Part model, mm, in its own coordinate system. Face numbers are marked on the shaded views. A direction names the side the tool comes from. Coordinates: 2 decimals unless noted, no trailing zeros. Order: outer loops, then holes, each group sorted by start corner. A loop starts at its lowest first (then second) coordinate and runs counter-clockwise, first axis right, second up. Notation, with made-up numbers: (-37, -12.5) - (4, -12.5) arc R29 cw to (4, 7.5) - close; hole circle Ø10 at (-3, 30.5). An arc over 180 degrees is marked (long way). Use a Markdown table: item, result. Add a question column.
1) Saw through at B-B on z = 0. List the corners of the cut face in (x, y), then the cut area to 3 significant figures.
2) Saw through at C-C on y = 12. List the corners of the cut face in (x, z), then the cut area to 3 significant figures.
3) Wall check: L1, parallel to Z at x = 0.1, y = 4; L2, parallel to X at y = 17, z = 2; L3, parallel to Y at x = -21.5, z = -4.5. Give the ranges that are in metal, low to high. Write a range as [from, to].
4) Tool access for the marked faces 1 and 2: list every direction of +Z, -Z, +X, -X, +Y, -Y with a clear straight run to the whole face (end or side of a thin tool).
5) Drop flat-ended pins along their axis: P1, Ø5, axis at x = -13, z = 0, coming from the -Y side; P2, Ø10, axis at x = -17, z = 9, coming from the +Y side; P3, Ø8.5, axis at y = 14.5, z = -5.5, coming from the -X side; P4, Ø12, axis at x = -25, y = 3.5, coming from the +Z side. Give the stop position or say it passes through.
6) Saw through at D-D on z = -3.5. List the corners of the cut face in (x, y), then the cut area to 3 significant figures.
7) Saw through at A-A on x = -13. List the corners of the cut face in (y, z), then the cut area to 3 significant figures.
```python
from build123d import *

# Parameters (mm, degrees)
BASE_FLANGE1_DEPTH       = 2
SKETCHED_START           = 1.372677549
SKETCHED_BEND1_OUTLINE_W = 2
SKETCHED_BEND1_OUTLINE_H = 30
SKETCHED_BEND1_DEPTH     = 28.627322451
SKETCHED_START_2         = -0.627322451
SKETCHED_BEND1_2_DEPTH   = 1.733838284
SKETCHED_START_3         = -1.363922451
SKETCHED_BEND1_3_DEPTH   = 2.7366
SKETCHED_START_4         = -15
SKETCHED_BEND1_4_DEPTH   = 30
SKETCH8_R                = 2
CUT_EXTRUDE1_DEPTH       = 10
SKETCH9_R                = 2
CUT_EXTRUDE2_DEPTH       = 10


with BuildPart() as part:
    # Base-Flange1: sheet metal written as solids
    # Sketch1 → Base-Flange1 (new body)
    with BuildSketch(Plane(origin=(0, 0, 0), x_dir=(1, 0, 0), z_dir=(0, 1, 0))):
        with BuildLine():
            Line((-20, -15), (20, -15))
            ThreePointArc((20, -15), (27.071067812, -12.071067812), (30, -5))
            Line((30, -5), (30, 5))
            ThreePointArc((30, 5), (27.071067812, 12.071067812), (20, 15))
            Line((20, 15), (-20, 15))
            ThreePointArc((-20, 15), (-27.071067812, 12.071067812), (-30, 5))
            Line((-30, 5), (-30, -5))
            ThreePointArc((-30, -5), (-27.071067812, -12.071067812), (-20, -15))
        make_face()
    extrude(amount=-BASE_FLANGE1_DEPTH)

    # Sketched Bend1: read off the stored shape, not the designer's step
    # Sketched Bend1 outline → Sketched Bend1 (cut)
    with BuildSketch(Plane.YZ.offset(SKETCHED_START)):
        with Locations((-1, 0)):
            Rectangle(SKETCHED_BEND1_OUTLINE_W, SKETCHED_BEND1_OUTLINE_H)
    extrude(amount=SKETCHED_BEND1_DEPTH, mode=Mode.SUBTRACT)

    # Sketched Bend1 2 outline → Sketched Bend1 2 (add)
    with BuildSketch(Plane.YZ.offset(SKETCHED_START_2)):
        with BuildLine():
            ThreePointArc((29.372677549, 5), (26.443745361, 12.071067812), (19.372677549, 15))
            Line((19.372677549, 15), (0, 15))
            Line((0, 15), (0, -15))
            Line((0, -15), (19.372677549, -15))
            ThreePointArc((19.372677549, -15), (26.443745361, -12.071067812), (29.372677549, -5))
            Line((29.372677549, -5), (29.372677549, 5))
        make_face()
    extrude(amount=SKETCHED_BEND1_2_DEPTH)

    # Sketched Bend1 3 outline → Sketched Bend1 3 (add)
    with BuildSketch(Plane.YZ.offset(SKETCHED_START_3)):
        with BuildLine():
            ThreePointArc((29.372677549, 5), (26.443745361, 12.071067812), (19.372677549, 15))
            Line((19.372677549, 15), (0, 15))
            Line((0, 15), (0, -15))
            Line((0, -15), (19.372677549, -15))
            ThreePointArc((19.372677549, -15), (26.443745361, -12.071067812), (29.372677549, -5))
            Line((29.372677549, -5), (29.372677549, 5))
        make_face()
    extrude(amount=SKETCHED_BEND1_3_DEPTH)

    # Sketched Bend1 4 outline → Sketched Bend1 4 (cut)
    with BuildSketch(Plane.XY.offset(SKETCHED_START_4)):
        with BuildLine():
            Line((-0.627322451, 0.7366), (-0.627322451, 29.372677549))
            Line((-0.627322451, 29.372677549), (-1.363922451, 29.372677549))
            Line((-1.363922451, 29.372677549), (-1.363922451, 0))
            ThreePointArc((-1.363922451, 0), (-0.843067596, 0.215745145), (-0.627322451, 0.7366))
        make_face()
        with BuildLine():
            Line((1.372677549, -2), (1.372677549, 0.7366))
            ThreePointArc((1.372677549, 0.7366), (0.571145967, -1.198468417), (-1.363922451, -2))
            Line((-1.363922451, -2), (1.372677549, -2))
        make_face()
    extrude(amount=SKETCHED_BEND1_4_DEPTH, mode=Mode.SUBTRACT)

    # Sketch8 → Cut-Extrude1 (cut)
    with BuildSketch(Plane.ZY.offset(0.627322451)):
        with Locations(Location((-8, 4, 0), (0, 0, 270))):
            Circle(SKETCH8_R)
        with Locations(Location((8, 4, 0), (0, 0, 270))):
            Circle(SKETCH8_R)
        with Locations(Location((-8, 12, 0), (0, 0, 270))):
            Circle(SKETCH8_R)
        with Locations(Location((-8, 20, 0), (0, 0, 270))):
            Circle(SKETCH8_R)
        with Locations(Location((8, 20, 0), (0, 0, 270))):
            Circle(SKETCH8_R)
        with Locations(Location((8, 12, 0), (0, 0, 270))):
            Circle(SKETCH8_R)
    extrude(amount=-CUT_EXTRUDE1_DEPTH, mode=Mode.SUBTRACT)

    # Sketch9 → Cut-Extrude2 (cut)
    with BuildSketch(Plane(origin=(0, 0, 0), x_dir=(1, 0, 0), z_dir=(0, 1, 0))):
        with Locations(Location((-23, 0, 0), (0, 0, 270))):
            Circle(SKETCH9_R)
        with Locations(Location((-13, 0, 0), (0, 0, 270))):
            Circle(SKETCH9_R)
    extrude(amount=-CUT_EXTRUDE2_DEPTH, mode=Mode.SUBTRACT)


solid = part.part
```
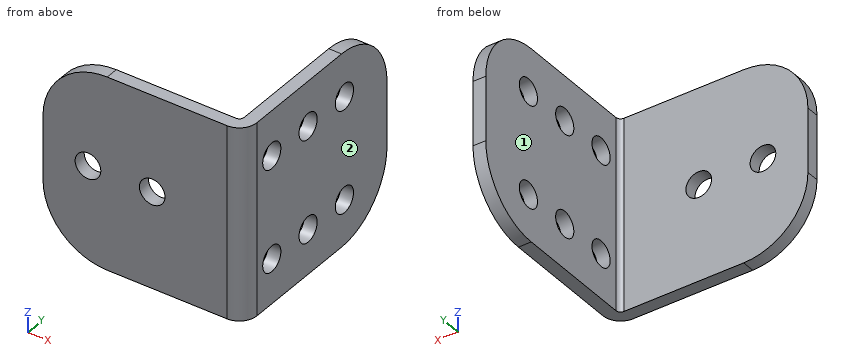
Results are:
| question | item | result |
|---|---|---|
| 1 | outline | (-30, -2) - (-25, -2) - (-25, 0) - (-30, 0) - close; (-21, -2) - (-15, -2) - (-15, 0) - (-21, 0) - close; (-11, -2) - (-1.36, -2) arc R2.74 ccw to (1.37, 0.74) - (1.37, 29.37) - (-0.63, 29.37) - (-0.63, 0.74) arc R0.74 cw to (-1.36, 0) - (-11, 0) - close |
| 1 | area | 104 mm2 |
| 2 | outline | (-0.63, -15) - (1.37, -15) - (1.37, -10) - (-0.63, -10) - close; (-0.63, -6) - (1.37, -6) - (1.37, 6) - (-0.63, 6) - close; (-0.63, 10) - (1.37, 10) - (1.37, 15) - (-0.63, 15) - close |
| 2 | area | 44.0 mm2 |
| 3 | L1 | [-15, -10], [-6, 6], [10, 15] |
| 3 | L2 | [-0.63, 1.37] |
| 3 | L3 | [-2, 0] |
| 4 | face 1 | +Z, -Z, -X, +Y |
| 4 | face 2 | +Z, -Z, +X, +Y, -Y |
| 5 | P1 | y = -2 |
| 5 | P2 | y = 0 |
| 5 | P3 | x = -0.63 |
| 5 | P4 | z = 15 |
| 6 | outline | (-30, -2) - (-1.36, -2) arc R2.74 ccw to (1.37, 0.74) - (1.37, 29.37) - (-0.63, 29.37) - (-0.63, 0.74) arc R0.74 cw to (-1.36, 0) - (-30, 0) - close |
| 6 | area | 120 mm2 |
| 7 | outline | (-2, -15) - (0, -15) - (0, -2) - (-2, -2) - close; (-2, 2) - (0, 2) - (0, 15) - (-2, 15) - close |
| 7 | area | 52.0 mm2 |
